Autodesk Inventor part; units mm, degrees
ref_plane "YZ Plane" through (0, 0, 0) normal (1, 0, 0) x (0, 1, 0)
ref_plane "XZ Plane" through (0, 0, 0) normal (0, 1, 0) x (-1, 0, 0)
ref_plane "XY Plane" through (0, 0, 0) normal (0, 0, 1) x (1, 0, 0)
sketch "スケッチ1" plane through (0, 0, 0) normal (0, 0, 1) x (1, 0, 0)
  line L0 (0, 0) -> (15, 0)
  line L1 (15, 0) -> (15, 15)
  line L2 (15, 15) -> (0, 15)
  line L3 (0, 15) -> (0, 0)
  dimension "d0" = 15
  dimension "d1" = 15
extrude "押し出し1" add sketch "スケッチ1" along normal blind 140
sketch "スケッチ3" plane through (0, 0, 0) normal (0, 0, -1) x (-1, 0, 0)
  line L0 (0, 0) -> (-15, 0)
  line L1 (-15, 0) -> (-15, 15)
  line L2 (-15, 15) -> (0, 15)
  line L3 (0, 15) -> (0, 0)
  dimension "d18" = 15
  dimension "d19" = 15
extrude "押し出し2" add sketch "スケッチ3" along normal blind 200
sketch "スケッチ4" plane through (0, 0, -200) normal (0, 0, -1) x (-1, 0, 0)
  point P0 (0, 0)
sketch "スケッチ6" plane through (0, 0, 140) normal (0, 0, 1) x (1, 0, 0)
  line L0 (0, 0) -> (0, 15)
  line L1 (15, 15) -> (15, 0)
  line L2 (0, 0) -> (15, 0)
  line L3 (15, 0) -> (15, 15)
  line L4 (15, 15) -> (0, 15)
  line L5 (0, 15) -> (0, 0)
extrude "押し出し3" cut sketch "スケッチ6" against normal blind 15
sketch "スケッチ8" plane through (0, 15, -200) normal (0, 1, 0) x (1, 0, 0)
  line L0 (0, 0) -> (15, 0)
  line L1 (15, 0) -> (15, -325)
  point P0 (0, -200)
  point P1 (7.5, -24)
  dimension "d36" = 24
  dimension "d37" = 7.5
hole "穴3" at (7.5, 15, -176) direction (0, -1, 0) diameter 3.2 end through all
sketch "スケッチ9" plane through (15, 0, -200) normal (1, 0, 0) x (0, 0, -1)
  line L0 (0, 15) -> (0, 0)
  line L1 (0, 15) -> (-325, 15)
  line L2 (-325, 0) -> (0, 0)
  point P0 (-200, 0)
  point P1 (-90, 7.5)
  point P2 (-100, 7.5)
  point P3 (-110, 7.5)
  point P4 (-150, 7.5)
  point P5 (-160, 7.5)
  point P6 (-170, 7.5)
  dimension "d45" = 90
  dimension "d46" = 7.5
  dimension "d47" = 10
  dimension "d48" = 10
  dimension "d49" = 7.5
  dimension "d50" = 7.5
  dimension "d51" = 40
  dimension "d52" = 7.5
  dimension "d53" = 10
  dimension "d54" = 7.5
  dimension "d55" = 10
  dimension "d56" = 7.5
hole "穴4" at (15, 7.5, -30) at (15, 7.5, -40) at (15, 7.5, -50) at (15, 7.5, -90) at (15, 7.5, -100) at (15, 7.5, -110) direction (-1, 0, 0) diameter 3.2 end through all
sketch "スケッチ10" plane through (0, 15, -200) normal (0, 1, 0) x (1, 0, 0)
  circle A0 centre (7.5, -24) radius 1.6
  line L0 (15, 0) -> (15, -325)
  point P0 (0, -200)
  point P1 (7.5, -34)
  dimension "d64" = 10
  dimension "d65" = 7.5
hole "穴5" at (7.5, 15, -166) direction (0, -1, 0) diameter 3.2 end through all
sketch "スケッチ11" plane through (0, 15, -200) normal (0, 1, 0) x (1, 0, 0)
  line L0 (0, -325) -> (15, -325)
  line L1 (15, 0) -> (15, -325)
  point P0 (0, -200)
  point P1 (7.5, -318)
  point P2 (7.5, -311)
  point P3 (7.5, -304)
  dimension "d73" = 7
  dimension "d74" = 7.5
  dimension "d75" = 7
  dimension "d76" = 7.5
  dimension "d77" = 7
  dimension "d78" = 7.5
hole "穴6" at (7.5, 15, 111) at (7.5, 15, 118) at (7.5, 15, 104) direction (0, -1, 0) diameter 3.2 end through all
sketch "スケッチ12" plane through (15, 0, -200) normal (1, 0, 0) x (0, 0, -1)
  line L0 (0, 15) -> (0, 0)
  line L1 (-325, 0) -> (0, 0)
  line L2 (0, 15) -> (-325, 15)
  point P0 (-200, 0)
  point P1 (-40, 7.5)
  point P2 (-50, 7.5)
  dimension "d86" = 40
  dimension "d87" = 7.5
  dimension "d88" = 7.5
  dimension "d89" = 10
hole "穴7" at (15, 7.5, -150) at (15, 7.5, -160) direction (-1, 0, 0) diameter 3.2 end through all
sketch "スケッチ13" plane through (0, 0, 125) normal (0, 0, 1) x (1, 0, 0)
  line L0 (1.5, 13.5) -> (13.5, 13.5)
  line L1 (13.5, 13.5) -> (13.5, 1.5)
  line L2 (13.5, 1.5) -> (1.5, 1.5)
  line L3 (1.5, 1.5) -> (1.5, 13.5)
  line L4 (0, 15) -> (15, 15)
  line L5 (0, 0) -> (0, 15)
  dimension "d97" = 12
  dimension "d98" = 12
  dimension "d99" = 1.5
  dimension "d100" = 1.5
extrude "押し出し4" cut sketch "スケッチ13" against normal blind 450
properties part number "射出_角柱4" material "アルミニウム 6061"
For this review, take the finished solid that the model builds, in its own axes (mm). A direction names the side the tool comes from. Coordinates: 2 decimals unless noted, no trailing zeros. Order: outer loops, then holes, each group sorted by start corner. A loop starts at its lowest first (then second) coordinate and runs counter-clockwise, first axis right, second up. Notation, with made-up numbers: (76.5, 40) -> (126.5, 40) arc R16 ccw to (126.5, 69) -> close; hole circle Ø10 at (12.25, 8.5). An arc over 180 degrees is marked (long way). Answer as CSV lines item,"result".
Q1. Wall thickness on line 1 along Z through (x, y) = (7.5, 14.15); line 2 along X through (y, z) = (8.75, 49): over which ranges is each line inside the solid? List them lowest first. Write a range as [from, to].
Model answer:
line 1,"z = [-200, -177.6], [-174.4, -167.6], [-164.4, 102.4], [105.6, 109.4], [112.6, 116.4], [119.6, 125]"
line 2,"x = [0, 1.5], [13.5, 15]"
Q2. For faces 5 (the face through (7, 0, -40)), 6 (the face through (8, 1.5, -35)), list the 3-axis set-ups (+Z, -Z, +X, -X, +Y, -Y) from which the entire face can be reached by the end or side of a thin tool; tool diameter is ignored.
Model answer:
face 5,"+Z, -Z, +X, -X, -Y"
face 6,"+Z, -Z"
Q3. Draft analysis for pull direction X (two halves, no side actions). For faces 1 (the face through (8, 15, -40)), 2 (the face through (0, 9.3, -39.8)), 3 (the face through (1.5, 7, -35)), 4 (the face through (15, 5.7, -39.8)), state which applies: released by +X, released by -X, zero draft, split by the parting line, or undercut.
Model answer:
face 1,"zero draft"
face 2,"released by -X"
face 3,"undercut"
face 4,"released by +X"
Q4. Clearance check with a flat-ended pin moving along its axis: pin 1 Ø2.5 at (y, z) = (7.5, -30) entering from -X (1 decimal). State where the tip first meets the part, or that it passes through.
Model answer:
pin 1,"passes through"
Q5. We need section A-A (z = -62). State the section outline as (x, y) points.
Model answer:
outline,"(0, 0) -> (15, 0) -> (15, 15) -> (0, 15) -> close; hole (1.5, 1.5) -> (13.5, 1.5) -> (13.5, 13.5) -> (1.5, 13.5) -> close"
